Part model, mm, in its own coordinate system. A direction names the side the tool comes from. Round coordinates to 2 decimals unless told otherwise and drop trailing zeros. Loops run counter-clockwise (first coordinate to the right, second up) from the corner with the lowest first, then second, coordinate; pieces in that order, holes last. Notation, with made-up numbers: M 74.5,-21.75 L 117.5,-21.75 A29 cw 117.5,4.25 Z; hole C -4.5,28.25 d5. An arc over 180 degrees is marked long. Write each question's results on one line, items separated by ' | '.
from build123d import *

# Parameters (mm, degrees)
F0_W          = 4.8315766917
F0_H          = 4.1204813641
F0_W_2        = 4.2928811043
F0_H_2        = 4.6790674097
F1_DEPTH      = 6.35
F1_DEPTH_BACK = 6.35
F2_DEPTH      = 6.35
F3_START      = 6.35
F3_DEPTH      = 8.89
F4_SIZE       = 0.254


# Not quite as in the source:
# - a feature names something its author has since deleted; it is built from what else it names


with BuildPart() as f1:
    # F0 (on Right) → F1 (new body, two sides)
    with BuildSketch(Plane.YZ) as f1_sk:
        with BuildLine():
            Line((0, -4.6790674097), (0, -6.35))
            ThreePointArc((0, -6.35), (1.9649498234, -6.0383335608), (3.7370149493, -5.1339282493))
            ThreePointArc((3.7370149493, -5.1339282493), (4.0213843703, -4.9143634121), (4.2928811043, -4.6790674097))
            Line((4.2928811043, -4.6790674097), (0, -4.6790674097))
        make_face()
        with BuildLine():
            Line((4.8315766917, -4.1204813641), (4.8315766917, 0))
            Line((4.8315766917, 0), (0, 0))
            Line((0, 0), (0, -4.6790674097))
            Line((0, -4.6790674097), (4.2928811043, -4.6790674097))
            ThreePointArc((4.2928811043, -4.6790674097), (4.5707698597, -4.4080112171), (4.8315766917, -4.1204813641))
        make_face()
        with Locations((2.4157883458, 2.0602406821)):
            Rectangle(F0_W, F0_H)
        with Locations((-2.1464405521, 2.0602406821)):
            Rectangle(F0_W_2, F0_H)
        with Locations((-2.1464405521, -2.3395337049)):
            Rectangle(F0_W_2, F0_H_2)
        with BuildLine():
            Line((-4.2928811043, 0), (-6.35, 0))
            ThreePointArc((-6.35, 0), (-5.813015354, -2.55565109), (-4.2928811043, -4.6790674097))
            Line((-4.2928811043, -4.6790674097), (-4.2928811043, 0))
        make_face()
        with BuildLine():
            ThreePointArc((-3.3540888173, -5.3919002407), (-1.7441234864, -6.105778678), (0, -6.35))
            Line((0, -6.35), (0, -4.6790674097))
            Line((0, -4.6790674097), (-4.2928811043, -4.6790674097))
            ThreePointArc((-4.2928811043, -4.6790674097), (-3.8400611852, -5.057314514), (-3.3540888173, -5.3919002407))
        make_face()
        with BuildLine():
            Line((4.8315766917, 0), (6.35, 0))
            ThreePointArc((6.35, 0), (5.958314023, 2.1956762065), (4.8315766917, 4.1204813641))
            Line((4.8315766917, 4.1204813641), (4.8315766917, 0))
        make_face()
        with BuildLine():
            ThreePointArc((4.8315766917, -4.1204813641), (5.958314023, -2.1956762065), (6.35, 0))
            Line((6.35, 0), (4.8315766917, 0))
            Line((4.8315766917, 0), (4.8315766917, -4.1204813641))
        make_face()
        with BuildLine():
            ThreePointArc((4.8315766917, 4.1204813641), (2.6605867151, 5.765741785), (0, 6.35))
            Line((0, 6.35), (0, 4.1204813641))
            Line((0, 4.1204813641), (4.8315766917, 4.1204813641))
        make_face()
        with BuildLine():
            Line((0, 4.1204813641), (0, 6.35))
            ThreePointArc((0, 6.35), (-4.4901280605, 4.4901280605), (-6.35, 0))
            Line((-6.35, 0), (-4.2928811043, 0))
            Line((-4.2928811043, 0), (-4.2928811043, 4.1204813641))
            Line((-4.2928811043, 4.1204813641), (0, 4.1204813641))
        make_face()
    extrude(amount=F1_DEPTH)
    extrude(f1_sk.sketch, amount=-F1_DEPTH_BACK)

    # F0 (on Right) → F2 (join)
    with BuildSketch(Plane.YZ):
        with BuildLine():
            ThreePointArc((0, -9.525), (6.7351920908, -6.7351920908), (9.525, 0))
            Line((9.525, 0), (6.35, 0))
            ThreePointArc((6.35, 0), (5.958314023, -2.1956762065), (4.8315766917, -4.1204813641))
            Line((4.8315766917, -4.1204813641), (4.8315766917, -4.6790674097))
            Line((4.8315766917, -4.6790674097), (4.2928811043, -4.6790674097))
            ThreePointArc((4.2928811043, -4.6790674097), (4.0213843703, -4.9143634121), (3.7370149493, -5.1339282493))
            ThreePointArc((3.7370149493, -5.1339282493), (1.9649498234, -6.0383335608), (0, -6.35))
            Line((0, -6.35), (0, -9.525))
        make_face()
        with BuildLine():
            Line((6.35, 0), (9.525, 0))
            ThreePointArc((9.525, 0), (6.7351920908, 6.7351920908), (0, 9.525))
            Line((0, 9.525), (0, 6.35))
            ThreePointArc((0, 6.35), (2.6605867151, 5.765741785), (4.8315766917, 4.1204813641))
            ThreePointArc((4.8315766917, 4.1204813641), (5.958314023, 2.1956762065), (6.35, 0))
        make_face()
        with BuildLine():
            Line((0, 6.35), (0, 9.525))
            ThreePointArc((0, 9.525), (-6.7351920908, 6.7351920908), (-9.525, 0))
            Line((-9.525, 0), (-6.35, 0))
            ThreePointArc((-6.35, 0), (-4.4901280605, 4.4901280605), (0, 6.35))
        make_face()
        with BuildLine():
            ThreePointArc((-9.525, 0), (-6.7351920908, -6.7351920908), (0, -9.525))
            Line((0, -9.525), (0, -6.35))
            ThreePointArc((0, -6.35), (-1.7441234864, -6.105778678), (-3.3540888173, -5.3919002407))
            ThreePointArc((-3.3540888173, -5.3919002407), (-3.8400611852, -5.057314514), (-4.2928811043, -4.6790674097))
            ThreePointArc((-4.2928811043, -4.6790674097), (-5.813015354, -2.55565109), (-6.35, 0))
            Line((-6.35, 0), (-9.525, 0))
        make_face()
    extrude(amount=F2_DEPTH)

    # F0 (on Right) → F3 (join)
    with BuildSketch(Plane.YZ.offset(F3_START)):
        with BuildLine():
            Line((4.8315766917, -4.1204813641), (4.8315766917, 0))
            Line((4.8315766917, 0), (0, 0))
            Line((0, 0), (0, -4.6790674097))
            Line((0, -4.6790674097), (4.2928811043, -4.6790674097))
            ThreePointArc((4.2928811043, -4.6790674097), (4.5707698597, -4.4080112171), (4.8315766917, -4.1204813641))
        make_face()
        with Locations((2.4157883458, 2.0602406821)):
            Rectangle(F0_W, F0_H)
        with Locations((-2.1464405521, 2.0602406821)):
            Rectangle(F0_W_2, F0_H)
        with Locations((-2.1464405521, -2.3395337049)):
            Rectangle(F0_W_2, F0_H_2)
    extrude(amount=F3_DEPTH)

    # F4
    f4_edges = [f1.edges().sort_by_distance(p)[0] for p in [
        (10.795, -4.292881, 4.120481),
        (10.795, -4.292881, -4.679067),
        (10.795, 4.831577, 4.120481),
    ]]
    chamfer(f4_edges, length=F4_SIZE)


solid = f1.part
Item 1: Band-saw the part on B-B on y = 5.5. Give the cut face in (x, z), and give its area (3 significant figures).
Filled sheet:
outline: M -6.35,-3.17 L 0,-3.17 L 0,-7.78 L 6.35,-7.78 L 6.35,7.78 L 0,7.78 L 0,3.17 L -6.35,3.17 Z | area: 139 mm^2
Item 2: Drop flat-ended pins along their axis: P1, Ø1.5, axis at x = 3.5, y = -2, coming from the +Z side; P2, Ø9, axis at x = 12.5, z = 0, coming from the -Y side; P3, Ø5, axis at x = 11.5, y = 6.5, coming from the +Z side. Give the stop position or say it passes through.
Filled sheet:
P1: z = 9.44 | P2: y = -4.29 | P3: z = 4.12
Item 3: Wall check: L1, parallel to Z at x = 11.5, y = 2.25; L2, parallel to X at y = -4.75, z = -1.75; L3, parallel to X at y = 5.5, z = 7.5. Give the ranges that are in metal, low to high.
Filled sheet:
L1: -4.68 to 4.12 | L2: -6.35 to 6.35 | L3: 0 to 6.35
Item 4: Band-saw the part on A-A on x = 4.25. Give the cut face in (y, z) (3 decimals), and give its area (3 significant figures).
Filled sheet:
outline: C 0,0 d19.05; hole M 4.293,-4.679 L 4.832,-4.679 L 4.832,-4.12 A6.35 cw Z | area: 285 mm^2
Item 5: Band-saw the part on D-D on z = 2.75. Give the cut face in (x, y).
Filled sheet:
outline: M -6.35,-5.72 L 0,-5.72 L 0,-9.12 L 6.35,-9.12 L 6.35,-4.29 L 15.24,-4.29 L 15.24,4.83 L 6.35,4.83 L 6.35,9.12 L 0,9.12 L 0,5.72 L -6.35,5.72 Z
Item 6: Band-saw the part on C-C on x = 13.5. Give the cut face in (y, z), and give its area (4 significant figures).
Filled sheet:
outline: M -4.29,-4.43 L -4.04,-4.68 L 4.29,-4.68 A6.35 ccw 4.83,-4.12 L 4.83,3.87 L 4.58,4.12 L -4.04,4.12 L -4.29,3.87 Z | area: 80.05 mm^2
Item 7: Which spindle directions (+Z, -Z, +X, -X, +Y, -Y) get a long thin tool onto all of the face, cutting with end or side? Do faces 1 (the flat face through (0, 6.2, -2)), 2 (the flat face through (11, 4.832, 0)), 3 (the flat face through (6.35, -0.1, 4.4)), 4 (the flat face through (11, 0, 4.12)). Say none if no direction does.
Filled sheet:
face 1: -X | face 2: +Z, -Z, +X, +Y | face 3: +X | face 4: +Z, +X, +Y, -Y
